The model under review builds one solid part; all positions refer to its coordinate system, in mm. A direction names the side the tool comes from. Round coordinates to 2 decimals unless told otherwise and drop trailing zeros. Write each loop counter-clockwise with the first axis right and the second up, starting at its lowest first coordinate (ties: lowest second). Pieces come first, ordered by that corner, then holes.
Item 1: Add section D-D (x = -27.38). Give the boundary of the cut face in (y, z), plus the area to 4 significant figures.
Item 2: Draft analysis for pull direction X (two halves, no side actions). For faces 3 (the face through (-50, -4, -31)), 4 (the face through (53, 4, 0)), 5 (the face through (52.377, -1.972, -30.542)), state which applies: +X half, -X half, draft (parallel to the pull), parting line (faces both ways), or undercut.
Item 3: To check wall thickness, follow L1, parallel to Y at x = -27, z = -22.5; L2, parallel to Y at x = -7.5, z = -3; L3, parallel to X at y = -2.75, z = 23. State the ranges of each line that lie inside material, in increasing order.
Item 4: Clearance check with flat-ended pins moving along their axes: pin 1 Ø6 at (x, z) = (0.5, -17) entering from -Y; pin 2 Ø10 at (x, z) = (14, 12.5) entering from +Y. State where each tip first meets the part, or that it passes through.
Item 5: Add section B-B (z = 24.5). Give the boundary of the cut face in (x, y), plus the area to 3 significant figures.
Item 6: Machinability: for faces 1 (the face through (-27.259, -1.972, 27.247)), 2 (the face through (50, -4, -31)), which of the approach directions +Z, -Z, +X, -X, +Y, -Y give a long, thin tool a straight path to every point of the face, cutting with its end or side? Answer none if there is none.
Item 7: Add section C-C (x = 49.65). Give the boundary of the cut face in (y, z), plus the area to 3 significant figures.
Item 8: Add section A-A (x = -9.5). Give the boundary of the cut face in (y, z), plus the area to 4 significant figures.
```python
from build123d import *

# Parameters (mm, degrees)
SKETCH1_W           = 106
SKETCH1_H           = 68
BOSS_EXTRUDE1_DEPTH = 8.5
SKETCH2_R           = 2.75
BOSS_EXTRUDE2_DEPTH = 4
SKETCH4_W           = 96
SKETCH4_H           = 55
CUT_EXTRUDE1_DEPTH  = 0.1


with BuildPart() as part:
    # Sketch1 → Boss-Extrude1 (new body)
    with BuildSketch(Plane(origin=(0, 0, 0), x_dir=(1, 0, 0), z_dir=(0, 1, 0))):
        Rectangle(SKETCH1_W, SKETCH1_H)
    extrude(amount=BOSS_EXTRUDE1_DEPTH)

    # Sketch2 → Boss-Extrude2 (add)
    with BuildSketch(Plane(origin=(0, 0, 0), x_dir=(-1, 0, 0), z_dir=(0, -1, 0))):
        with Locations(Location((49.65, -30.9, 0), (0, 0, 90))):
            Circle(SKETCH2_R)
        with Locations(Location((-49.65, -30.9, 0), (0, 0, 90))):
            Circle(SKETCH2_R)
        with Locations(Location((49.65, 30.9, 0), (0, 0, 90))):
            Circle(SKETCH2_R)
        with Locations(Location((-49.65, 30.9, 0), (0, 0, 90))):
            Circle(SKETCH2_R)
        with Locations(Location((27.38, -24.5, 0), (0, 0, 90))):
            Circle(SKETCH2_R)
        with Locations(Location((-30.62, -24.5, 0), (0, 0, 90))):
            Circle(SKETCH2_R)
        with Locations(Location((27.38, 24.54, 0), (0, 0, 90))):
            Circle(SKETCH2_R)
        with Locations(Location((-30.62, 24.54, 0), (0, 0, 90))):
            Circle(SKETCH2_R)
    extrude(amount=BOSS_EXTRUDE2_DEPTH)

    # Sketch4 → Cut-Extrude1 (cut)
    with BuildSketch(Plane(origin=(0, 8.5, 0), x_dir=(1, 0, 0), z_dir=(0, 1, 0))):
        with Locations((0, -2.5)):
            Rectangle(SKETCH4_W, SKETCH4_H)
    extrude(amount=-CUT_EXTRUDE1_DEPTH, mode=Mode.SUBTRACT)


solid = part.part
```
Numbers:
1. outline: (-4, -27.29) - (0, -27.29) - (0, -34) - (8.5, -34) - (8.5, -25) - (8.4, -25) - (8.4, 30) - (8.5, 30) - (8.5, 34) - (0, 34) - (0, 27.25) - (-4, 27.25) - (-4, 21.75) - (0, 21.75) - (0, -21.79) - (-4, -21.79) - close
1. area: 616.5 mm2
2. face 3: draft
2. face 4: +X half
2. face 5: undercut
3. L1: y = -4 to 8.4
3. L2: y = 0 to 8.4
3. L3: x = -29.68 to -25.08, 28.32 to 32.92
4. pin 1: stops at y = 0
4. pin 2: stops at y = 8.4
5. outline: (-53, 0) - (-30.13, 0) - (-30.13, -4) - (-24.63, -4) - (-24.63, 0) - (27.87, 0) - (27.87, -4) - (33.37, -4) - (33.37, 0) - (53, 0) - (53, 8.5) - (48, 8.5) - (48, 8.4) - (-48, 8.4) - (-48, 8.5) - (-53, 8.5) - close
5. area: 935 mm2
6. face 1: -Y
6. face 2: +Z, -Z, +X, -X, -Y
7. outline: (-4, -33.65) - (0, -33.65) - (0, -34) - (8.5, -34) - (8.5, 34) - (0, 34) - (0, 33.65) - (-4, 33.65) - (-4, 28.15) - (0, 28.15) - (0, -28.15) - (-4, -28.15) - close
7. area: 622 mm2
8. outline: (0, -34) - (8.5, -34) - (8.5, -25) - (8.4, -25) - (8.4, 30) - (8.5, 30) - (8.5, 34) - (0, 34) - close
8. area: 572.5 mm2
